```python
from build123d import *
from OCP.BRepFilletAPI import BRepFilletAPI_MakeFillet

# Parameters (mm, degrees)
SKETCH1_W           = 6
SKETCH1_H           = 6
BOSS_EXTRUDE1_DEPTH = 1.5
SKETCH5_W           = 6
SKETCH5_H           = 6
BOSS_EXTRUDE2_DEPTH = 3
SKETCH2_W           = 4
SKETCH2_H           = 4
CUT_EXTRUDE1_DEPTH  = 2
SKETCH10_W          = 4
SKETCH10_H          = 1.5
CUT_EXTRUDE3_DEPTH  = 9.717797887
FILLET7_R1          = 0.5
FILLET7_R2          = 1.5


with BuildPart() as part:
    # Sketch1 → Boss-Extrude1 (new, symmetric)
    with BuildSketch(Plane.XY):
        with Locations((3, 3)):
            Rectangle(SKETCH1_W, SKETCH1_H)
        with Locations((-3, 3)):
            Rectangle(SKETCH1_W, SKETCH1_H)
    extrude(amount=BOSS_EXTRUDE1_DEPTH, both=True)

    # Sketch5 → Boss-Extrude2 (add)
    with BuildSketch(Plane.XY.offset(1.5)):
        with Locations((0, -3)):
            Rectangle(SKETCH5_W, SKETCH5_H)
    extrude(amount=-BOSS_EXTRUDE2_DEPTH)

    # Sketch2 → Cut-Extrude1 (cut)
    with BuildSketch(Plane.XY.offset(1.5)):
        with Locations((3, 3)):
            Rectangle(SKETCH2_W, SKETCH2_H)
        with Locations((-3, 3)):
            Rectangle(SKETCH2_W, SKETCH2_H)
        with Locations((0, -3)):
            Rectangle(SKETCH2_W, SKETCH2_H)
    extrude(amount=-CUT_EXTRUDE1_DEPTH, mode=Mode.SUBTRACT)

    # Sketch10 → Cut-Extrude3 (cut, through all)
    with BuildSketch(Plane.XY.offset(-0.5)):
        with Locations((0, -3)):
            Rectangle(SKETCH10_W, SKETCH10_H)
        with Locations((3, 3)):
            Rectangle(SKETCH10_W, SKETCH10_H)
        with Locations((-3, 3)):
            Rectangle(SKETCH10_W, SKETCH10_H)
    extrude(amount=-CUT_EXTRUDE3_DEPTH, mode=Mode.SUBTRACT)

    # Fillet7: one fillet with a radius per group of edges: ONE call of the kernel's fillet builder (fillet() takes one radius for all edges)
    fillet7_edges_1 = [part.edges().sort_by_distance(p)[0] for p in [
        (6, 0, 0),
        (3, -6, 0),
        (6, 6, 0),
        (-6, 6, 0),
        (-6, 0, 0),
        (-3, -6, 0),
    ]]
    fillet7_edges_2 = [part.edges().sort_by_distance(p)[0] for p in [
        (3, 0, 0),
        (-3, 0, 0),
    ]]
    fillet7 = BRepFilletAPI_MakeFillet(part.part.solid().wrapped)
    for e in fillet7_edges_1:
        fillet7.Add(FILLET7_R1, e.wrapped)
    for e in fillet7_edges_2:
        fillet7.Add(FILLET7_R2, e.wrapped)
    add(Compound.cast(fillet7.Shape()), mode=Mode.REPLACE)


solid = part.part
```
Part model, mm, in its own coordinate system. A direction names the side the tool comes from. Give positions to 0.01 mm unless a question says otherwise; leave off trailing zeros. Order: outer loops, then holes, each group sorted by start corner. A loop starts at its lowest first (then second) coordinate and runs counter-clockwise, first axis right, second up. Notation, with made-up numbers: (10, 20) - (23, 20) arc R20 ccw to (23, 33) - close; hole circle Ø2 at (87, 43.25). An arc over 180 degrees is marked (long way). Use one line per item in the form item = value.
Item 1: Two-plate mould, pull along X, no slides. Class faces 5 (the face through (3, -4, 0)), 6 (the face through (-6, 3, 0)), 7 (the face through (3, 3.75, -1)): released by +X, released by -X, zero draft, split by the parting line, or undercut.
Solution:
face_5 = released by +X
face_6 = released by -X
face_7 = undercut
Item 2: Slice it at B-B on z = -1.2. Give the cut face in (x, y), and give its area (3 significant figures).
Solution:
outline = (-6, 0.5) arc R0.5 ccw to (-5.5, 0) - (-4.5, 0) arc R1.5 cw to (-3, -1.5) - (-3, -5.5) arc R0.5 ccw to (-2.5, -6) - (2.5, -6) arc R0.5 ccw to (3, -5.5) - (3, -1.5) arc R1.5 cw to (4.5, 0) - (5.5, 0) arc R0.5 ccw to (6, 0.5) - (6, 5.5) arc R0.5 ccw to (5.5, 6) - (-5.5, 6) arc R0.5 ccw to (-6, 5.5) - close; hole (-5, 2.25) - (-1, 2.25) - (-1, 3.75) - (-5, 3.75) - close; hole (-2, -3.75) - (2, -3.75) - (2, -2.25) - (-2, -2.25) - close; hole (1, 2.25) - (5, 2.25) - (5, 3.75) - (1, 3.75) - close
area = 90.6 mm2
Item 3: Probe probe 1 along Y at (x, z) = (1.25, -0.4); probe 2 along Y at (x, z) = (0.5, -1.35). List the from-to ranges inside material, lowest first. Write a range as from..to.
Solution:
probe_1 = -6..-5, -1..1, 5..6
probe_2 = -6..-3.75, -2.25..6
Item 4: Slice it at A-A on x = 4.75. Give the cut face in (y, z), and give its area (3 significant figures).
Solution:
outline = (0, -1.5) - (2.25, -1.5) - (2.25, -0.5) - (1, -0.5) - (1, 1.5) - (0, 1.5) - close; (3.75, -1.5) - (6, -1.5) - (6, 1.5) - (5, 1.5) - (5, -0.5) - (3.75, -0.5) - close
area = 8.50 mm2
Item 5: Slice it at D-D on y = 1.75. Give the cut face in (x, z).
Solution:
outline = (-6, -1.5) - (6, -1.5) - (6, 1.5) - (5, 1.5) - (5, -0.5) - (1, -0.5) - (1, 1.5) - (-1, 1.5) - (-1, -0.5) - (-5, -0.5) - (-5, 1.5) - (-6, 1.5) - close
Item 6: Pin check, flat tips, straight feed: pin 1 Ø1 at (x, z) = (-4, 1) entering from -Y; pin 2 Ø1.5 at (x, z) = (-4, 0.5) entering from -Y; pin 3 Ø0.6 at (x, y) = (3, 1.5) entering from +Z; pin 4 Ø1.1 at (x, z) = (-3, -1) entering from -Y. Stop position of each tip, or through.
Solution:
pin_1 = -0.38
pin_2 = -0.67
pin_3 = -0.5
pin_4 = -6
Item 7: Slice it at C-C on x = -1.75. Give the cut face in (y, z), and give its area (3 significant figures).
Solution:
outline = (-6, -1.5) - (-3.75, -1.5) - (-3.75, -0.5) - (-5, -0.5) - (-5, 1.5) - (-6, 1.5) - close; (-2.25, -1.5) - (2.25, -1.5) - (2.25, -0.5) - (1, -0.5) - (1, 1.5) - (-1, 1.5) - (-1, -0.5) - (-2.25, -0.5) - close; (3.75, -1.5) - (6, -1.5) - (6, 1.5) - (5, 1.5) - (5, -0.5) - (3.75, -0.5) - close
area = 17.0 mm2
Item 8: Which spindle directions (+Z, -Z, +X, -X, +Y, -Y) get a long thin tool onto all of the face, cutting with end or side? Do faces 1 (the face through (3, 5, 1)), 2 (the face through (-3, -4, 0)), 3 (the face through (0, -2.25, -1)), 4 (the face through (3.45, -0.43, -0.02)). Say none if no direction does.
Solution:
face_1 = +Z
face_2 = +Z, -Z, -X, -Y
face_3 = +Z, -Z
face_4 = +Z, -Z, +X, -Y
